Autodesk Inventor part; units mm, degrees
ref_plane "YZ Plane" through (0, 0, 0) normal (1, 0, 0) x (0, 1, 0)
ref_plane "XZ Plane" through (0, 0, 0) normal (0, 1, 0) x (-1, 0, 0)
ref_plane "XY Plane" through (0, 0, 0) normal (0, 0, 1) x (1, 0, 0)
sketch "スケッチ1" plane through (0, 0, 0) normal (0, 0, 1) x (1, 0, 0)
  line L0 (-35, 25) -> (35, 25)
  line L1 (35, 25) -> (35, -25)
  line L2 (35, -25) -> (-35, -25)
  line L3 (-35, -25) -> (-35, 25)
  line L4 (-35, 25) -> (35, -25) construction
  line L5 (35, 25) -> (-35, -25) construction
  point P0 (0, 0)
  dimension "d0" = 70
  dimension "d1" = 50
extrude "押し出し1" add sketch "スケッチ1" along normal blind 1.5
sketch "スケッチ2" plane through (0, 0, 1.5) normal (0, 0, 1) x (1, 0, 0)
  line L0 (-25, 25) -> (25, 25)
  line L1 (25, 25) -> (25, -15)
  line L2 (25, -15) -> (-25, -15)
  line L3 (-25, -15) -> (-25, 25)
  line L4 (-35, 25) -> (-35, -25)
  line L5 (35, -25) -> (35, 25)
  line L6 (-35, -25) -> (35, -25)
  point P0 (0, 0)
  dimension "d4" = 10
  dimension "d5" = 10
  dimension "d6" = 10
extrude "押し出し2" cut sketch "スケッチ2" against normal blind 1.5
sketch "スケッチ3" plane through (0, 0, 1.5) normal (0, 0, 1) x (1, 0, 0)
  line L0 (35, -25) -> (35, 25)
  line L1 (-35, 25) -> (-35, -25)
  line L2 (25, -15) -> (-25, -15)
  point P0 (0, 0)
  point P1 (-17.5, -20)
  point P2 (17.5, -20)
  dimension "d9" = 17.5
  dimension "d10" = 17.5
  dimension "d11" = 5
hole "穴1" at (-17.5, -20, 1.5) at (17.5, -20, 1.5) direction (0, 0, -1) diameter 3.1 end through all
sketch "スケッチ5" plane through (0, 0, 1.5) normal (0, 0, 1) x (1, 0, 0)
  line L0 (-35, -25) -> (35, -25)
  line L1 (-35, 25) -> (-35, -25)
  point P0 (0, 0)
  point P1 (-5, -20)
  point P2 (5, -20)
  point P3 (-35, 55)
  dimension "d21" = 10
  dimension "d22" = 5
  dimension "d23" = 30
hole "穴2" at (-5, -20, 1.5) at (5, -20, 1.5) direction (0, 0, -1) diameter 3.1 end through all
sketch "スケッチ6" plane through (0, 0, 1.5) normal (0, 0, 1) x (1, 0, 0)
  line L0 (0, 82.7836) -> (64.7866, 82.7836)
  line L1 (64.7866, 82.7836) -> (64.7866, -43.11)
  line L2 (64.7866, -43.11) -> (0, -43.11)
  line L3 (0, -43.11) -> (0, 82.7836)
  point P0 (0, 0)
extrude "押し出し4" cut sketch "スケッチ6" against normal blind 30
sketch "スケッチ7" plane through (-35, 25, 1.5) normal (0, 1, 0) x (1, 0, 0)
  line L0 (0, 0) -> (10, 0)
  line L1 (10, 0) -> (10, 1.5)
  line L2 (10, 1.5) -> (0, 1.5)
  line L3 (0, 1.5) -> (0, 0)
  point P0 (35, 1.5)
extrude "押し出し5" add sketch "スケッチ7" along normal blind 30
properties part number "爪_4" material "アルミニウム 6061"
Geometry: final body of the model. Coordinates: model frame, mm. A direction names the side the tool comes from. Round coordinates to 2 decimals unless told otherwise and drop trailing zeros. Order: outer loops, then holes, each group sorted by start corner. A loop starts at its lowest first (then second) coordinate and runs counter-clockwise, first axis right, second up. Notation, with made-up numbers: (-37, 47) -> (-16, 47) arc R15 cw to (-16, 69) -> close; hole circle Ø10 at (-12.75, 73). An arc over 180 degrees is marked (long way). Put each result on its own line as item: value. Start each with the question number.
Q1. Reachability of faces 1 (the flat face through (-17, -25, 1)), 2 (the flat face through (-12, -15, 1)) from +Z, -Z, +X, -X, +Y, -Y: full face, straight path, thin tool, end or side. Return the list, or none.
Q2. First-contact query: pin 1 (0.8 mm diameter, centred on x = -14, z = 1, fed in from +Y). Flat tip, straight axial feed; report the tip coordinate or a pass-through.
Q3. Section C-C on y = -20. Return the cut outline in (x, z).
Q4. Section A-A on x = -17.5. Return the cut outline in (y, z).
Q5. Section D-D on x = -23. Return the cut outline in (y, z).
Q6. Pull-direction query (Y, two-part tool) for faces 3 (the cylindrical face through (-4.406, -21.432, 0.74)), 4 (the flat face through (-30, 55, 1)), 5 (the cylindrical face through (-18.81, -20.83, 0.74)), 6 (the flat face through (-25, 20, 1)); classes: +Y half, -Y half, draft (parallel to the pull), parting line (faces both ways), or undercut.
Q7. Section B-B on z = 0.8. Return the cut outline in (x, y).
Q8. Line query: probe 1 along X at (y, z) = (-20, 1.1); probe 2 along Y at (x, z) = (-5, 0.6); probe 3 along X at (y, z) = (42, 1.3). Output: solid intervals per line, ascending.
Ans:
1. face 1: +Z, -Z, +X, -X, -Y
1. face 2: +Z, -Z, +X, +Y
2. pin 1: stops at y = -15
3. outline: (-35, 0) -> (-19.05, 0) -> (-19.05, 1.5) -> (-35, 1.5) -> close; (-15.95, 0) -> (-6.55, 0) -> (-6.55, 1.5) -> (-15.95, 1.5) -> close; (-3.45, 0) -> (0, 0) -> (0, 1.5) -> (-3.45, 1.5) -> close
4. outline: (-25, 0) -> (-21.55, 0) -> (-21.55, 1.5) -> (-25, 1.5) -> close; (-18.45, 0) -> (-15, 0) -> (-15, 1.5) -> (-18.45, 1.5) -> close
5. outline: (-25, 0) -> (-15, 0) -> (-15, 1.5) -> (-25, 1.5) -> close
6. face 3: undercut
6. face 4: +Y half
6. face 5: undercut
6. face 6: draft
7. outline: (-35, -25) -> (0, -25) -> (0, -15) -> (-25, -15) -> (-25, 55) -> (-35, 55) -> close; hole circle Ø3.1 at (-17.5, -20); hole circle Ø3.1 at (-5, -20)
8. probe 1: x = -35 to -19.05, -15.95 to -6.55, -3.45 to 0
8. probe 2: y = -25 to -21.55, -18.45 to -15
8. probe 3: x = -35 to -25
